Check sheet for the modelled part. Datum: model origin and axes. Units: mm. A direction names the side the tool comes from. Coordinates: 2 decimals unless noted, no trailing zeros. Write each loop counter-clockwise with the first axis right and the second up, starting at its lowest first coordinate (ties: lowest second). Pieces come first, ordered by that corner, then holes. Notation, with made-up numbers: (16.25, 4) -> (58.25, 4) arc R22 cw to (58.25, 41) -> close; hole circle Ø5 at (-39.5, -22.5). An arc over 180 degrees is marked (long way). Put each result on its own line as item: value.
```python
from build123d import *

# Parameters (mm, degrees)
SZKIC1_R                    = 50
DODANIE_WYCI_GNI_CIE1_DEPTH = 5
SZKIC2_R                    = 17.5
DODANIE_WYCI_GNI_CIE2_DEPTH = 120
OTW_R_POD_RUB_M81_D         = 9


with BuildPart() as part:
    # Szkic1 → Dodanie-wyciągnięcie1 (new body)
    with BuildSketch(Plane(origin=(0, 0, 0), x_dir=(1, 0, 0), z_dir=(0, 1, 0))):
        with Locations(Location((0, 0, 0), (0, 0, 270))):
            Circle(SZKIC1_R)
    extrude(amount=DODANIE_WYCI_GNI_CIE1_DEPTH)

    # Szkic2 → Dodanie-wyciągnięcie2 (add)
    with BuildSketch(Plane(origin=(0, 5, 0), x_dir=(1, 0, 0), z_dir=(0, 1, 0))):
        with Locations(Location((0, 0, 0), (0, 0, 270))):
            Circle(SZKIC2_R)
    extrude(amount=DODANIE_WYCI_GNI_CIE2_DEPTH)

    # Otwór pod śrubę M81 (through all)
    with Locations(Plane(origin=(0, 5, 0), x_dir=(1, 0, 0), z_dir=(0, 1, 0))):
        with Locations((-33.75, 0), (0, 33.75), (0, -33.75), (33.75, 0)):
            Hole(OTW_R_POD_RUB_M81_D / 2)


solid = part.part
```
Q1. Cross-section at A-A (x = 0). Record the cut outline in (y, z), plus the area to 3 significant figures.
Recorded:
outline: (0, -50) -> (5, -50) -> (5, -38.25) -> (0, -38.25) -> close; (0, -29.25) -> (5, -29.25) -> (5, -17.5) -> (125, -17.5) -> (125, 17.5) -> (5, 17.5) -> (5, 29.25) -> (0, 29.25) -> close; (0, 38.25) -> (5, 38.25) -> (5, 50) -> (0, 50) -> close
area: 4,610 mm2
Q2. Depth check by flat-ended pin: P1, Ø4, axis at x = 34, z = -39.5, coming from the -Y side (3 decimals); P2, Ø14.5, axis at x = -33.75, z = 0, coming from the +Y side; P3, Ø4, axis at y = 93.5, z = -9, coming from the +X side; P4, Ø1.5, axis at y = 38.5, z = -5, coming from the -X side. Enter the tip coordinate at first touch or a pass-through.
Recorded:
P1: passes through
P2: stops at y = 5
P3: stops at x = 16.04
P4: stops at x = -16.98
Q3. Material ranges on line 1 along Y through (x, z) = (28, -2); line 2 along X through (y, z) = (1, -33); line 3 along X through (y, z) = (24.5, 0), recorded low to high.
Recorded:
line 1: y = 0 to 5
line 2: x = -37.56 to -4.44, 4.44 to 37.56
line 3: x = -17.5 to 17.5
Q4. Tool access check on faces 1 (the cylindrical face through (-10.648, 64.16, -13.887)), 2 (the cylindrical face through (0.98, 2.47, -29.36)). Record the directions out of +Z, -Z, +X, -X, +Y, -Y that give a thin tool (end or side, any length) a straight path to the whole face; none if there is none.
Recorded:
face 1: +Y
face 2: +Y, -Y
Q5. Cross-section at C-C (z = 33.75). Record the cut outline in (x, y).
Recorded:
outline: (-36.89, 0) -> (-4.5, 0) -> (-4.5, 5) -> (-36.89, 5) -> close; (4.5, 0) -> (36.89, 0) -> (36.89, 5) -> (4.5, 5) -> close
Q6. Cross-section at B-B (z = 0). Record the cut outline in (x, y), plus the area to 3 significant figures.
Recorded:
outline: (-50, 0) -> (-38.25, 0) -> (-38.25, 5) -> (-50, 5) -> close; (-29.25, 0) -> (29.25, 0) -> (29.25, 5) -> (17.5, 5) -> (17.5, 125) -> (-17.5, 125) -> (-17.5, 5) -> (-29.25, 5) -> close; (38.25, 0) -> (50, 0) -> (50, 5) -> (38.25, 5) -> close
area: 4,610 mm2
Q7. Cross-section at D-D (x = -33.75). Record the cut outline in (y, z).
Recorded:
outline: (0, -36.89) -> (5, -36.89) -> (5, -4.5) -> (0, -4.5) -> close; (0, 4.5) -> (5, 4.5) -> (5, 36.89) -> (0, 36.89) -> close
Q8. Mould release check, pull along X, two halves, no side actions. Record for faces 3 (the cylindrical face through (0.98, 2.47, 38.14)), 4 (the cylindrical face through (15.02, 2.46, 47.69)), 5 (the flat face through (1, 0, -1)): released by +X, released by -X, zero draft, split by the parting line, or undercut.
Recorded:
face 3: undercut
face 4: split by the parting line
face 5: zero draft
